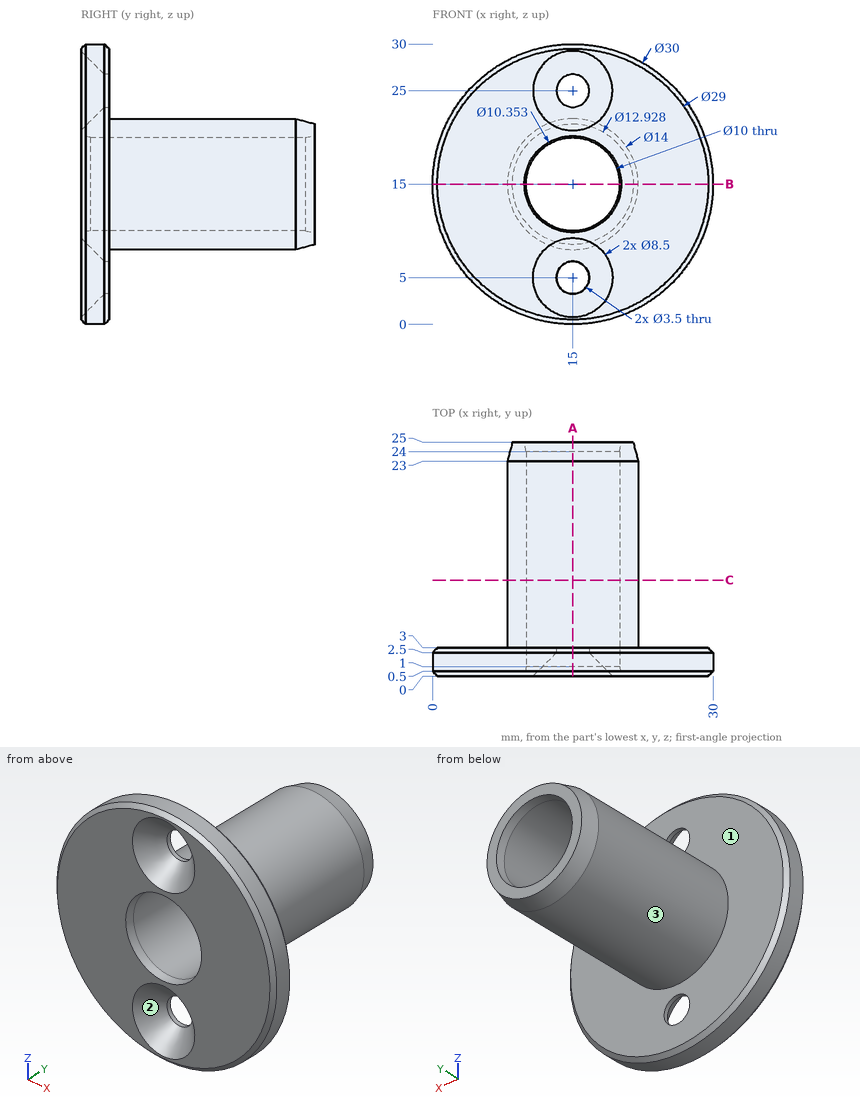
Study the drawing (mm; zero at the part's minimum x, y, z) and answer. Give positions to 0.01 mm unless a question says otherwise; leave off trailing zeros. Order: outer loops, then holes, each group sorted by start corner. A loop starts at its lowest first (then second) coordinate and runs counter-clockwise, first axis right, second up. Notation, with made-up numbers: (-26, 49) - (13, 49) arc R20 cw to (13, 87) - close; hole circle Ø3 at (83, -18.75). An arc over 180 degrees is marked (long way). Answer as CSV lines item,"result". Start each with the question number.
Q1. Find the intervals of material crossed by L1, parallel to X at y = 11.5, z = 15; L2, parallel to Y at x = 19.25, z = 21.5; L3, parallel to Z at x = 11.75, y = 8.75, in increasing order. Write a range as [from, to].
Q2. The part is cut by section A-A (x = 15). Give the number of separate pieces and of enclosed holes in the cut face.
Q3. The part is cut by section C-C (y = 10.25). Write down the section's boundary in (x, z).
Q4. Given pin 1 Ø10 at (y, z) = (13.5, 23.5) entering from -X; pin 2 Ø2 at (x, y) = (19, 18.5) entering from +Z (1 decimal); pin 3 Ø6 at (x, y) = (24, 4.5) entering from -Z; pin 4 Ø3 at (x, z) = (15, 25) entering from +Y, each flat-ended and moving along its own axis, determine where each tip first touches the part or whether it passes through.
Q5. The part is cut by section B-B (z = 15). Write down the section's boundary in (x, y).
Q6. The mould has two halves that part along X. Classify the marked faces 1, 2 and 3: +X half, -X half, draft (parallel to the pull), parting line (faces both ways), or undercut.
Check result:
1,L1,"x = [8, 10], [20, 22]"
1,L2,"y = [0, 3]"
1,L3,"z = [8.8, 11.2], [18.8, 21.2]"
2,separate pieces,"4"
2,enclosed holes,"0"
3,outline,"circle Ø14 at (15, 15); hole circle Ø10 at (15, 15)"
4,pin 1,"stops at x = 8.94"
4,pin 2,"stops at z = 21.3"
4,pin 3,"stops at z = 1.61"
4,pin 4,"passes through"
5,outline,"(0, 0.5) - (0.5, 0) - (9.82, 0) - (10, 1) - (10, 24) - (9.82, 25) - (8.54, 25) - (8, 23) - (8, 3) - (0.5, 3) - (0, 2.5) - close; (20, 1) - (20.18, 0) - (29.5, 0) - (30, 0.5) - (30, 2.5) - (29.5, 3) - (22, 3) - (22, 23) - (21.46, 25) - (20.18, 25) - (20, 24) - close"
6,face 1,"draft"
6,face 2,"undercut"
6,face 3,"parting line"
